```python
from build123d import *

# Parameters (mm, degrees)
SKETCH1_R               = 4.7625
SKETCH1_R_2             = 4.1275
SHAFTBODY_DEPTH         = 127
SIDECUTS_DEPTH          = 128.178468353
SIDECUTS_DEPTH_BACK     = 128.178468353
CUT_EXTRUDE2_REACH      = 129.178
CUT_EXTRUDE2_END_RADIUS = 4.7625


with BuildPart() as part:
    # Sketch1 → ShaftBody (new body)
    with BuildSketch(Plane.XY):
        Circle(SKETCH1_R)
        Circle(SKETCH1_R_2, mode=Mode.SUBTRACT)
    extrude(amount=-SHAFTBODY_DEPTH)

    # Sketch6 → SideCuts (cut, two sides: drawn at the far end of the back side and taken through both)
    with BuildSketch(Plane(origin=(0, 0, 0), x_dir=(0, 0, -1), z_dir=(1, 0, 0)).offset(-SIDECUTS_DEPTH_BACK)):
        with BuildLine():
            Line((6.0325, 1.5875), (0, 1.5875))
            Line((0, 1.5875), (0, -1.5875))
            Line((0, -1.5875), (6.0325, -1.5875))
            ThreePointArc((6.0325, -1.5875), (7.62, 0), (6.0325, 1.5875))
        make_face()
    extrude(amount=SIDECUTS_DEPTH + SIDECUTS_DEPTH_BACK, mode=Mode.SUBTRACT)

    # Cut-Extrude2: up to this cylinder (the profile starts inside it)
    cut_extrude2_end = Plane(origin=(0, 0, -10.16), z_dir=(0, 0, 1)) * Cylinder(CUT_EXTRUDE2_END_RADIUS, 268.881, mode=Mode.PRIVATE)
    # Sketch7 → Cut-Extrude2 (cut, up to the surface)
    with BuildSketch(Plane(origin=(0, 0, 0), x_dir=(1, 0, 0), z_dir=(0, 1, 0)), mode=Mode.PRIVATE) as cut_extrude2_sk1:
        with BuildLine():
            Line((-0.635, 3.81), (0.635, 3.81))
            ThreePointArc((0.635, 3.81), (1.084012806, 3.995987194), (1.27, 4.445))
            Line((1.27, 4.445), (1.27, 15.875))
            ThreePointArc((1.27, 15.875), (1.084012806, 16.324012806), (0.635, 16.51))
            Line((0.635, 16.51), (-0.635, 16.51))
            ThreePointArc((-0.635, 16.51), (-1.084012806, 16.324012806), (-1.27, 15.875))
            Line((-1.27, 15.875), (-1.27, 4.445))
            ThreePointArc((-1.27, 4.445), (-1.084012806, 3.995987194), (-0.635, 3.81))
        make_face()
    cut_extrude2_tool1 = extrude(cut_extrude2_sk1.sketch, amount=CUT_EXTRUDE2_REACH, mode=Mode.PRIVATE) & cut_extrude2_end
    add(cut_extrude2_tool1.solids().sort_by_distance((0, 0, -10.16))[0], mode=Mode.SUBTRACT)


solid = part.part
```
For this review, take the finished solid that the model builds, in its own axes (mm). Round coordinates to 2 decimals unless told otherwise and drop trailing zeros. Write each loop counter-clockwise with the first axis right and the second up, starting at its lowest first coordinate (ties: lowest second). Pieces come first, ordered by that corner, then holes. Notation, with made-up numbers: (-21.75, 48) - (14.25, 48) arc R16 cw to (14.25, 77) - close; hole circle Ø5 at (-35.5, 40). An arc over 180 degrees is marked (long way). Use CSV: the item, a comma, the result in double quotes.
1) Clearance check with flat-ended pins moving along their axes: pin 1 Ø5 at (x, z) = (3.5, -97.5) entering from +Y; pin 2 Ø0.5 at (y, z) = (4.5, -8) entering from -X; pin 3 Ø0.7 at (x, z) = (-4, -3) entering from -Y. State where each tip first meets the part, or that it passes through.
Conclusion:
pin 1,"stops at y = 4.66"
pin 2,"stops at x = -2.15"
pin 3,"stops at y = -3.06"
2) Wall thickness on line 1 along X through (y, z) = (0, -75.5); line 2 along Y through (x, z) = (0.25, -119); line 3 along Y through (x, z) = (-3.5, -60): over which ranges is each line inside the solid? List them lowest first. Write a range as from..to.
Conclusion:
line 1,"x = -4.76..-4.13, 4.13..4.76"
line 2,"y = -4.76..-4.12, 4.12..4.76"
line 3,"y = -3.23..-2.19, 2.19..3.23"
3) Add section C-C on z = -21. Write out the cut boundary in (x, y) (1 decimal).
Conclusion:
outline,"circle Ø9.5 at (0, 0); hole circle Ø8.3 at (0, 0)"
4) Add section B-B on y = 0. Write out the cut boundary in (x, z), and give its area (3 significant figures).
Conclusion:
outline,"(-4.76, -127) - (-4.13, -127) - (-4.13, -7.62) - (-4.76, -7.62) - close; (4.13, -127) - (4.76, -127) - (4.76, -7.62) - (4.13, -7.62) - close"
area,"152 mm^2"
5) The part is to be moulded in two halves that separate along Y. For faces 1 (the flat face through (-4, 2, -127)), 2 (the cylindrical face through (-3.275, -2.512, -62.611)), 3 (the cylindrical face through (-1.03, -4.65, -62.61)), say which applies: pulls with the +Y half, pulls with the -Y half, needs draft (parallel to the pull), parting line crosses it, or undercut.
Conclusion:
face 1,"needs draft"
face 2,"undercut"
face 3,"parting line crosses it"
6) Add section A-A on x = -2.75. Write out the cut boundary in (y, z), and give its area (3 significant figures).
Conclusion:
outline,"(-3.89, -127) - (-3.08, -127) - (-3.08, 0) - (-3.89, 0) - close; (3.08, -127) - (3.89, -127) - (3.89, 0) - (3.08, 0) - close"
area,"206 mm^2"
